The figure shows three views and two pictorial views of one solid part (mm, origin at its lowest corner). Answer the questions. A direction names the side the tool comes from. Round coordinates to 2 decimals unless told otherwise and drop trailing zeros. Loops run counter-clockwise (first coordinate to the right, second up) from the corner with the lowest first, then second, coordinate; pieces in that order, holes last. Notation, with made-up numbers: (5, -33.5) -> (52, -33.5) arc R8 ccw to (52, -24.5) -> close; hole circle Ø8 at (-35, -5.5). An arc over 180 degrees is marked (long way). Write item = value, one per line. Start each with the question number.
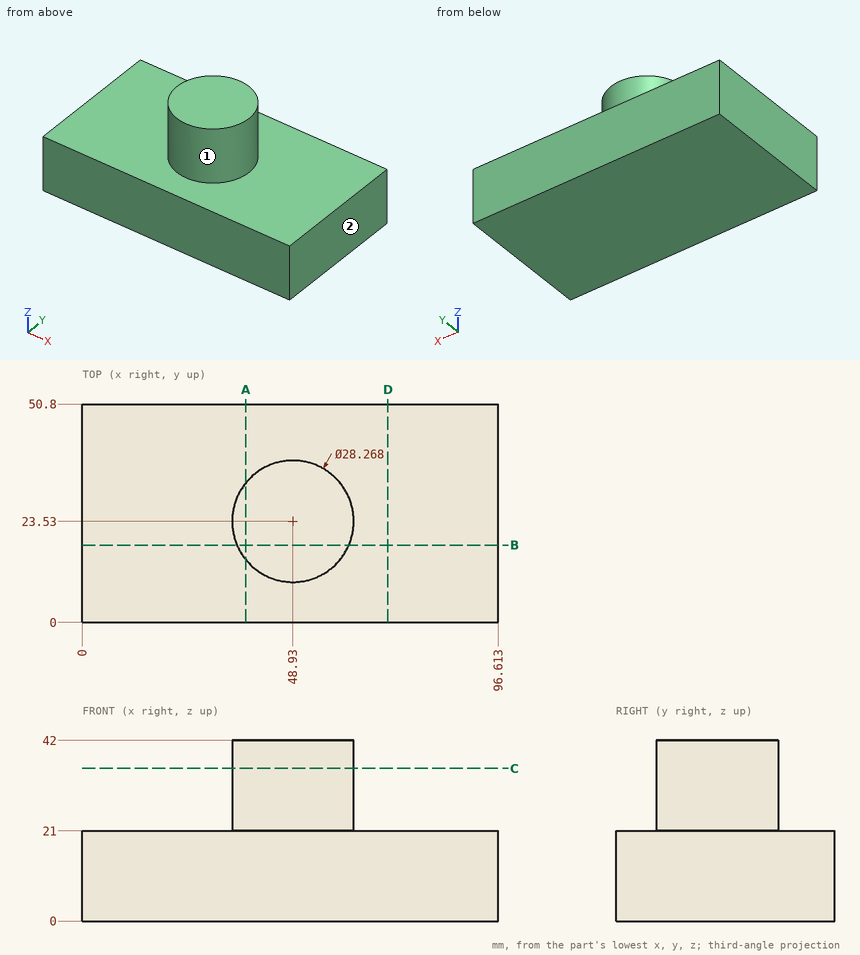
Item 1: Section B-B (y = 18) is taken. Determine the outline of the cut face in (x, z).
Item 2: Section A-A (x = 38) is taken. Determine the outline of the cut face in (y, z), then the cut area to 3 significant figures.
Item 3: Find the intervals of material crossed by line 1 along Z through (x, y) = (15, 33.5); line 2 along X through (y, z) = (23, 27) (1 decimal); line 3 along X through (y, z) = (35, 30.5), in increasing order. Write a range as [from, to].
Item 4: Section D-D (x = 71) is taken. Determine the outline of the cut face in (y, z).
Item 5: Flat-ended cylindrical pins translate along their axes: pin 1 (2 mm diameter, centred on y = 45.5, z = 19.5, fed in from -X); pin 2 (15 mm diameter, centred on x = 71.5, y = 23, fed in from +Z); pin 3 (1 mm diameter, centred on y = 25.5, z = 37, fed in from -X). Find the tip coordinate at first contact, or state that the pin passes through.
Item 6: Section C-C (z = 35.5) is taken. Determine the outline of the cut face in (x, y) (1 decimal).
Item 7: A tool of negligible diameter and unlimited length cuts with its end or side. For the marked faces 1 and 2, from which of +Z, -Z, +X, -X, +Y, -Y can it reach the whole face along a straight path? Write none if from no direction.
Worked answers:
q1.outline = (0, 0) -> (96.61, 0) -> (96.61, 21) -> (61.94, 21) -> (61.94, 42) -> (35.92, 42) -> (35.92, 21) -> (0, 21) -> close
q2.outline = (0, 0) -> (50.8, 0) -> (50.8, 21) -> (32.49, 21) -> (32.49, 42) -> (14.57, 42) -> (14.57, 21) -> (0, 21) -> close
q2.area = 1,440 mm2
q3.line_1 = [0, 21]
q3.line_2 = [34.8, 63.1]
q3.line_3 = [40.67, 57.19]
q4.outline = (0, 0) -> (50.8, 0) -> (50.8, 21) -> (0, 21) -> close
q5.pin_1 = 0
q5.pin_2 = 21
q5.pin_3 = 34.87
q6.outline = circle Ø28.3 at (48.9, 23.5)
q7.face_1 = +Z
q7.face_2 = +Z, -Z, +X, +Y, -Y
